```python
from build123d import *

# Parameters (mm, degrees)
CROQUIS1_W     = 30
CROQUIS1_H     = 40
CROQUIS1_H_2   = 30
CROQUIS1_W_2   = 40
EXTRUIR1_DEPTH = 30
CROQUIS5_W     = 30
CROQUIS5_H     = 30
EXTRUIR4_DEPTH = 40
CROQUIS8_W     = 30
CROQUIS8_H     = 30
EXTRUIR6_DEPTH = 40
CROQUIS9_W     = 30
CROQUIS9_H     = 30
CROQUIS9_W_2   = 24
CROQUIS9_H_2   = 24
EXTRUIR7_DEPTH = 40
CROQUIS2_W     = 30
CROQUIS2_H     = 30
CROQUIS2_W_2   = 24
CROQUIS2_H_2   = 24
EXTRUIR2_DEPTH = 40
CROQUIS3_W     = 30
CROQUIS3_H     = 30
CROQUIS3_W_2   = 24
CROQUIS3_H_2   = 24
EXTRUIR3_DEPTH = 40
CROQUIS7_W     = 30
CROQUIS7_H     = 30
CROQUIS7_W_2   = 24
CROQUIS7_H_2   = 24
EXTRUIR5_DEPTH = 40
VACIADO1_T     = -2


with BuildPart() as part:
    # Croquis1 → Extruir1 (new body)
    with BuildSketch(Plane(origin=(0, 0, 0), x_dir=(1, 0, 0), z_dir=(0, 1, 0))):
        with Locations((0, 35)):
            Rectangle(CROQUIS1_W, CROQUIS1_H)
        Rectangle(CROQUIS1_W, CROQUIS1_H_2)
        with Locations((35, 0)):
            Rectangle(CROQUIS1_W_2, CROQUIS1_H_2)
    extrude(amount=EXTRUIR1_DEPTH)

    # Croquis5 → Extruir4 (add)
    with BuildSketch(Plane.XZ):
        Rectangle(CROQUIS5_W, CROQUIS5_H)
    extrude(amount=EXTRUIR4_DEPTH)

    # Croquis8 → Extruir6 (add)
    with BuildSketch(Plane(origin=(0, 30, 0), x_dir=(1, 0, 0), z_dir=(0, 1, 0))):
        Rectangle(CROQUIS8_W, CROQUIS8_H)
    extrude(amount=EXTRUIR6_DEPTH)

    # Croquis9 → Extruir7 (cut)
    with BuildSketch(Plane(origin=(0, 70, 0), x_dir=(1, 0, 0), z_dir=(0, 1, 0))):
        Rectangle(CROQUIS9_W, CROQUIS9_H)
        Rectangle(CROQUIS9_W_2, CROQUIS9_H_2, mode=Mode.SUBTRACT)
    extrude(amount=-EXTRUIR7_DEPTH, mode=Mode.SUBTRACT)

    # Croquis2 → Extruir2 (cut)
    with BuildSketch(Plane(origin=(55, 0, 0), x_dir=(0, 0, -1), z_dir=(1, 0, 0))):
        with Locations((0, 15)):
            Rectangle(CROQUIS2_W, CROQUIS2_H)
        with Locations((0, 15)):
            Rectangle(CROQUIS2_W_2, CROQUIS2_H_2, mode=Mode.SUBTRACT)
    extrude(amount=-EXTRUIR2_DEPTH, mode=Mode.SUBTRACT)

    # Croquis3 → Extruir3 (cut)
    with BuildSketch(Plane(origin=(0, 0, -55), x_dir=(-1, 0, 0), z_dir=(0, 0, -1))):
        with Locations((0, 15)):
            Rectangle(CROQUIS3_W, CROQUIS3_H)
        with Locations((0, 15)):
            Rectangle(CROQUIS3_W_2, CROQUIS3_H_2, mode=Mode.SUBTRACT)
    extrude(amount=-EXTRUIR3_DEPTH, mode=Mode.SUBTRACT)

    # Croquis7 → Extruir5 (cut)
    with BuildSketch(Plane.XZ.offset(40)):
        Rectangle(CROQUIS7_W, CROQUIS7_H)
        Rectangle(CROQUIS7_W_2, CROQUIS7_H_2, mode=Mode.SUBTRACT)
    extrude(amount=-EXTRUIR5_DEPTH, mode=Mode.SUBTRACT)

    # Vaciado1
    vaciado1_openings = [part.faces().sort_by_distance(p)[0] for p in [
        (0, 15, -55),
        (0, -40, 0),
        (0, 70, 0),
        (55, 15, 0),
    ]]
    offset(amount=VACIADO1_T, openings=vaciado1_openings, kind=Kind.INTERSECTION)


solid = part.part
```
For this review, take the finished solid that the model builds, in its own axes (mm). A direction names the side the tool comes from. Round coordinates to 2 decimals unless told otherwise and drop trailing zeros. Write each loop counter-clockwise with the first axis right and the second up, starting at its lowest first coordinate (ties: lowest second). Pieces come first, ordered by that corner, then holes. Notation, with made-up numbers: (-27, 40) -> (-12, 40) arc R38 ccw to (-12, 79) -> close; hole circle Ø3 at (55, -26.5). An arc over 180 degrees is marked (long way). Use one line per item in the form item = value.
Q1. Consider section C-C (x = 38.5). State the section outline as (y, z) points, then the cut area to 3 significant figures.
Resolved:
outline = (3, -12) -> (27, -12) -> (27, 12) -> (3, 12) -> close; hole (5, -10) -> (25, -10) -> (25, 10) -> (5, 10) -> close
area = 176 mm²
Q2. Consider section B-B (y = 31.5). State the section outline as (x, z) points.
Resolved:
outline = (-12, -12) -> (12, -12) -> (12, 12) -> (-12, 12) -> close; hole (-10, -10) -> (10, -10) -> (10, 10) -> (-10, 10) -> close
Q3. To check wall thickness, follow probe 1 along Y at (x, z) = (36, -8); probe 2 along Z at (x, y) = (4, -32). State the ranges of each line that lie inside material, in increasing order. Write a range as from..to.
Resolved:
probe_1 = 3..5, 25..27
probe_2 = -12..-10, 10..12
Q4. Clearance check with flat-ended pins moving along their axes: pin 1 Ø7 at (y, z) = (43.5, 2.5) entering from -X; pin 2 Ø7 at (x, y) = (2.5, -16.5) entering from +Z; pin 3 Ø12 at (x, z) = (32, 0) entering from -Y; pin 4 Ø10 at (x, y) = (21, -26.5) entering from -Z. State where each tip first meets the part, or that it passes through.
Resolved:
pin_1 = -12
pin_2 = 12
pin_3 = 3
pin_4 = through
Q5. Consider section A-A (z = -3.5). State how many separate pieces and enclosed holes the cut face has, then the cut area to 3 significant figures.
Resolved:
separate_pieces = 3
enclosed_holes = 0
area = 584 mm²
Q6. The part is to be moulded in two halves that separate along X. For faces 5 (the flat face through (-14, 15, -15)), 6 (the flat face through (12, 15, -35)), 7 (the flat face through (0, 25, -34)), 8 (the flat face through (-12, 28, 0)), say which applies: released by +X, released by -X, zero draft, split by the parting line, or undercut.
Resolved:
face_5 = zero draft
face_6 = released by +X
face_7 = undercut
face_8 = undercut
Q7. Machinability: for faces 1 (the flat face through (35, 27, 0)), 2 (the flat face through (0, 27, -35)), 3 (the flat face through (34, 15, 10)), 4 (the flat face through (10, 49, 0)), which of the approach directions +Z, -Z, +X, -X, +Y, -Y give a long, thin tool a straight path to every point of the face, cutting with its end or side? Answer none if there is none.
Resolved:
face_1 = +Z, -Z, +X, +Y
face_2 = -Z, +X, -X, +Y
face_3 = +X
face_4 = +Y, -Y
